Source: CAD feature listing. Evaluate the final solid. Frame: model axes, mm. A direction names the side the tool comes from. Coordinates: 2 decimals unless noted, no trailing zeros. Order: outer loops, then holes, each group sorted by start corner. A loop starts at its lowest first (then second) coordinate and runs counter-clockwise, first axis right, second up.
```python
from build123d import *

# Parameters (mm, degrees)
SKETCH_W     = 42
SKETCH_H     = 42
PAD_DEPTH    = 20
SKETCH001_R  = 7
PAD001_DEPTH = 4.5
SKETCH002_R  = 3
HOLE_DEPTH   = 0.5
HOLE_TIPS_R  = 3
SKETCH003_W  = 23.5
SKETCH003_H  = 5.5
POCKET_DEPTH = 5


with BuildPart() as part:
    # Sketch → Pad (new body)
    with BuildSketch(Plane.XZ):
        with Locations((8.147526, -9.378734)):
            Rectangle(SKETCH_W, SKETCH_H)
    extrude(amount=PAD_DEPTH)

    # Sketch001 (on Face5 of Pad) → Pad001 (join)
    with BuildSketch(Plane(origin=(0, 0, 0), x_dir=(1, 0, 0), z_dir=(0, 1, 0))):
        with Locations((8.142856, 9.219142)):
            Circle(SKETCH001_R)
    extrude(amount=PAD001_DEPTH)

    # Sketch002 (on Face8 of Pad001) → Hole (cut)
    with BuildSketch(Plane(origin=(0, 4.5, 0), x_dir=(1, 0, 0), z_dir=(0, 1, 0))):
        with Locations((8.27745, 9.219093)):
            Circle(SKETCH002_R)
    extrude(amount=-HOLE_DEPTH, mode=Mode.SUBTRACT)

    # Hole tips → Hole tip 1 section 0
    with BuildSketch(Plane(origin=(0, 4, 0), x_dir=(1, 0, 0), z_dir=(0, 1, 0)), mode=Mode.PRIVATE) as hole_tip_1_s0:
        with Locations((8.27745, 9.219093)):
            Circle(HOLE_TIPS_R)
    loft([hole_tip_1_s0.sketch, Vertex(8.27745, 2.197418, -9.219093)], mode=Mode.SUBTRACT)

    # Sketch003 (on Face5 of Hole) → Pocket (cut)
    with BuildSketch(Plane.XZ.offset(20)):
        with Locations((8.721823, -22.801634)):
            Rectangle(SKETCH003_W, SKETCH003_H)
    extrude(amount=-POCKET_DEPTH, mode=Mode.SUBTRACT)


solid = part.part
```
Q1. Set-up query: faces 5 (the cylindrical face through (9.662, 4.254, -6.558)), 6 (the flat face through (9, -15, -23)), 7 (the flat face through (8, 4.5, -6)). Return all of +Z, -Z, +X, -X, +Y, -Y with unobstructed straight access to the full face (end or side cutting, diameter ignored); none if empty.
Solutions:
face 5: +Y
face 6: -Y
face 7: +Z, -Z, +X, -X, +Y
Q2. Material intervals for line 1 along Z through (x, y) = (14, -17); line 2 along Y through (x, z) = (8, -24); line 3 along Y through (x, z) = (2.5, -14.5), sorted ascending.
Solutions:
line 1: z = -30.38 to -25.55, -20.05 to 11.62
line 2: y = -15 to 0
line 3: y = -20 to 0
Q3. Pin query (flat end, axial travel): P1, Ø1.5, axis at x = 17, z = -8.5, coming from the +Y side; P2, Ø4.5, axis at x = 11.5, z = -23, coming from the -Y side. Return the tip coordinate at first contact, or that it passes through.
Solutions:
P1: stops at y = 0
P2: stops at y = -15
Q4. Section query A-A on z = -13.5. Output: boundary loops of the cut face in (x, y), plus the area to 3 significant figures.
Solutions:
outline: (-12.85, -20) - (29.15, -20) - (29.15, 0) - (13.68, 0) - (13.68, 4.5) - (2.6, 4.5) - (2.6, 0) - (-12.85, 0) - close
area: 890 mm2
Q5. Section query B-B on x = 19.5. Output: boundary loops of the cut face in (y, z), plus the area to 4 significant figures.
Solutions:
outline: (-20, -30.38) - (0, -30.38) - (0, 11.62) - (-20, 11.62) - (-20, -20.05) - (-15, -20.05) - (-15, -25.55) - (-20, -25.55) - close
area: 812.5 mm2
Q6. Section query C-C on y = 3. Output: boundary loops of the cut face in (x, z), plus the area to 3 significant figures.
Solutions:
outline: circle Ø14 at (8.14, -9.22); hole circle Ø2.67 at (8.28, -9.22)
area: 148 mm2
Q7. Section query D-D on z = 0.5. Output: boundary loops of the cut face in (x, y).
Solutions:
outline: (-12.85, -20) - (29.15, -20) - (29.15, 0) - (-12.85, 0) - close
Q8. Pull-direction query (Z, two-part tool) for faces 1 (the flat face through (-3.028, -18, -23)), 2 (the cylindrical face through (14.82, 2.22, -11.32)), 3 (the flat face through (8, -10, 11.621)), 4 (the flat face through (8, -20, -9)); classes: pulls with the +Z half, pulls with the -Z half, needs draft (parallel to the pull), parting line crosses it, or undercut.
Solutions:
face 1: undercut
face 2: parting line crosses it
face 3: pulls with the +Z half
face 4: needs draft
